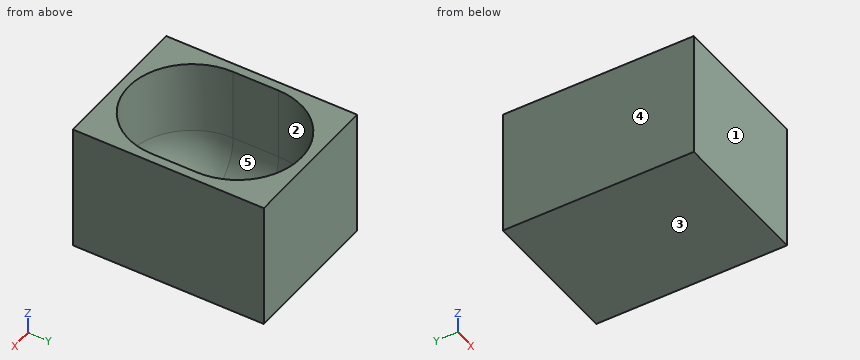
from build123d import *

# Parameters (mm, degrees)
SKETCH019_W     = 16
SKETCH019_H     = 21
PAD005_DEPTH    = 14
POCKET012_DEPTH = 13
FILLET001_R     = 5


with BuildPart() as part:
    # Sketch019 → Pad005 (new body)
    with BuildSketch(Plane.XY):
        with Locations((-67.67703, 154.469096)):
            Rectangle(SKETCH019_W, SKETCH019_H)
    extrude(amount=PAD005_DEPTH)

    # Sketch020 (on Face6 of Pad005) → Pocket012 (cut)
    with BuildSketch(Plane.XY.offset(14)):
        with BuildLine():
            ThreePointArc((-60.67703, 156.969096), (-67.67703, 163.969096), (-74.67703, 156.969096))
            Line((-74.67703, 156.969096), (-74.67703, 151.969096))
            ThreePointArc((-74.67703, 151.969096), (-67.67703, 144.969096), (-60.67703, 151.969096))
            Line((-60.67703, 156.969096), (-60.67703, 151.969096))
        make_face()
    extrude(amount=-POCKET012_DEPTH, mode=Mode.SUBTRACT)

    # Fillet001
    fillet001_edges = [part.edges().sort_by_distance(p)[0] for p in [
        (-67.67703, 144.969096, 1),
        (-74.67703, 154.469096, 1),
        (-60.67703, 154.469096, 1),
        (-67.67703, 163.969096, 1),
    ]]
    fillet(fillet001_edges, radius=FILLET001_R)


solid = part.part
Source: CAD feature listing. Evaluate the final solid. Frame: model axes, mm. Face numbers are marked on the shaded views. A direction names the side the tool comes from. Coordinates: 2 decimals unless noted, no trailing zeros. Order: outer loops, then holes, each group sorted by start corner. A loop starts at its lowest first (then second) coordinate and runs counter-clockwise, first axis right, second up. Notation, with made-up numbers: M -38,-28.5 L 3,-28.5 A15 ccw 3,-24.5 Z; hole C 5.5,12 d4. An arc over 180 degrees is marked long. Write each question's results on one line, items separated by ' | '. Start each with the question number.
1. Section A-A, the plane z = 12.75. Return the cut outline in (x, y).
2. Material intervals for L1, parallel to X at y = 152, z = 12.5; L2, parallel to Z at x = -67.5, y = 155.25; L3, parallel to X at y = 159.5, z = 12, sorted ascending.
3. Section B-B, the plane y = 154. Return the cut outline in (x, z), then the cut area to 3 significant figures.
4. Reachability of the marked faces 1 and 2 from +Z, -Z, +X, -X, +Y, -Y: full face, straight path, thin tool, end or side. Return the list, or none.
5. Draft query along X for the marked faces 3, 4 and 5. Return one class per face: +X half, -X half, draft (parallel to the pull), parting line (faces both ways), or undercut.
6. Pin query (flat end, axial travel): pin 1 (3 mm diameter, centred on x = -68.5, y = 155.5, fed in from +Z). Return the tip coordinate at first contact, or that it passes through.
Solution:
1) outline: M -75.68,143.97 L -59.68,143.97 L -59.68,164.97 L -75.68,164.97 Z; hole M -74.68,151.97 A7 ccw -60.68,151.97 L -60.68,156.97 A7 ccw -74.68,156.97 Z
2) L1: -75.68 to -74.68, -60.68 to -59.68 | L2: 0 to 1 | L3: -75.68 to -74.2, -61.15 to -59.68
3) outline: M -75.68,0 L -59.68,0 L -59.68,14 L -60.68,14 L -60.68,6 A5 cw -65.68,1 L -69.68,1 A5 cw -74.68,6 L -74.68,14 L -75.68,14 Z | area: 52.7 mm²
4) face 1: +Z, -Z, +X, -X, -Y | face 2: +Z
5) face 3: draft | face 4: -X half | face 5: undercut
6) pin 1: z = 1.01
